Autodesk Inventor part; units mm, degrees
ref_plane "Work Plane1" through (0, 0, 0) normal (0, 0, 1) x (1, 0, 0)
ref_plane "YZ Plane" through (0, 0, 0) normal (1, 0, 0) x (0, 1, 0)
ref_plane "XZ Plane" through (0, 0, 0) normal (0, 1, 0) x (-1, 0, 0)
ref_plane "Work Plane1" through (0, 0, 0) normal (0, 0, 1) x (1, 0, 0)
sketch "Sketch1" plane through (0, 0, 0) normal (0, 0, 1) x (1, 0, 0)
  line L0 (302, -174.3598) -> (0, -348.7196)
  line L1 (0, -348.7196) -> (-302, -174.3598)
  line L2 (-302, -174.3598) -> (-302, 174.3598)
  line L3 (-302, 174.3598) -> (0, 348.7196)
  line L4 (0, 348.7196) -> (302, 174.3598)
  line L5 (302, 174.3598) -> (302, -174.3598)
  line L6 (498, -287.5204) -> (0, -575.0409)
  line L7 (0, -575.0409) -> (-498, -287.5204)
  line L8 (-498, -287.5204) -> (-498, 287.5204)
  line L9 (-498, 287.5204) -> (0, 575.0409)
  line L10 (0, 575.0409) -> (498, 287.5204)
  line L11 (498, 287.5204) -> (498, -287.5204)
  point P0 (0, 0)
  point P1 (0, 0)
  point P2 (0, 0)
  dimension "d0" = 302
  dimension "d1" = 498
extrude "Extrusion1" add sketch "Sketch1" along normal blind 10
properties part number "Membrane" material "Nylon 6/6"
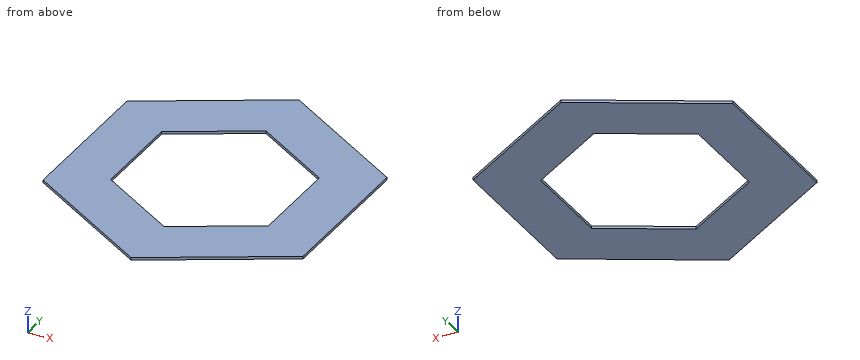
For this review, take the finished solid that the model builds, in its own axes (mm). Give positions to 0.01 mm unless a question says otherwise; leave off trailing zeros. Write each loop counter-clockwise with the first axis right and the second up, starting at its lowest first coordinate (ties: lowest second). Pieces come first, ordered by that corner, then holes.
Item 1: Take a section at C-C (x = 184.5). Give the boundary of the cut face in (y, z).
Item 2: Wall thickness on probe 1 along X at (y, z) = (-29, 1.75); probe 2 along Y at (x, z) = (94.5, 3); probe 3 along X at (y, z) = (-233, 1.5): over which ranges is each line inside the solid? List them lowest first.
Item 3: Insertion check: P1, Ø5, axis at x = 71, z = 6, coming from the -Y side; P2, Ø6, axis at y = -378, z = 5, coming from the -X side; P3, Ø5, axis at x = 42, z = 8.5, coming from the -Y side. Each pin has a flat end and moves straight along its axis. Give the tip position at first contact, or say it passes through.
Item 4: Take a section at B-B (y = -23.5). Give the boundary of the cut face in (x, z).
Item 5: Take a section at A-A (z = 8.5). Give the boundary of the cut face in (x, y), and give its area (3 significant figures).
Item 6: Take a section at D-D (y = -449). Give the boundary of the cut face in (x, z), and give its area (3 significant figures).
Established:
1. outline: (-468.52, 0) - (-242.2, 0) - (-242.2, 10) - (-468.52, 10) - close; (242.2, 0) - (468.52, 0) - (468.52, 10) - (242.2, 10) - close
2. probe 1: x = -498 to -302, 302 to 498
2. probe 2: y = -520.48 to -294.16, 294.16 to 520.48
2. probe 3: x = -498 to -200.43, 200.43 to 498
3. P1: stops at y = -535.49
3. P2: stops at x = -346.48
3. P3: stops at y = -552.24
4. outline: (-498, 0) - (-302, 0) - (-302, 10) - (-498, 10) - close; (302, 0) - (498, 0) - (498, 10) - (302, 10) - close
5. outline: (-498, -287.52) - (0, -575.04) - (498, -287.52) - (498, 287.52) - (0, 575.04) - (-498, 287.52) - close; hole (-302, -174.36) - (0, -348.72) - (302, -174.36) - (302, 174.36) - (0, 348.72) - (-302, 174.36) - close
5. area: 543,000 mm2
6. outline: (-218.31, 0) - (218.31, 0) - (218.31, 10) - (-218.31, 10) - close
6. area: 4,370 mm2
